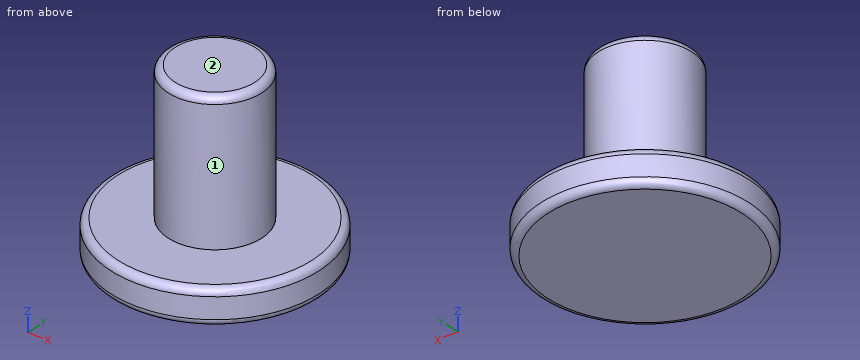
```python
from build123d import *

# Parameters (mm, degrees)
F0_R     = 6.75
F1_DEPTH = 25
F0_R_2   = 15
F2_DEPTH = 5
F3_R     = 1


with BuildPart() as f1:
    # F0 (on Top) → F1 (new body)
    with BuildSketch(Plane.XY):
        Circle(F0_R)
    extrude(amount=F1_DEPTH)

    # F0 (on Top) → F2 (join)
    with BuildSketch(Plane.XY):
        Circle(F0_R_2)
        Circle(F0_R, mode=Mode.SUBTRACT)
    extrude(amount=F2_DEPTH)

    # F3
    f3_edges = [f1.edges().sort_by_distance(p)[0] for p in [
        (-15, 0, 0),
        (-15, 0, 5),
        (-6.75, 0, 25),
    ]]
    fillet(f3_edges, radius=F3_R)


solid = f1.part
```
For this review, take the finished solid that the model builds, in its own axes (mm). Face numbers are marked on the shaded views. A direction names the side the tool comes from. Round coordinates to 2 decimals unless told otherwise and drop trailing zeros. Write each loop counter-clockwise with the first axis right and the second up, starting at its lowest first coordinate (ties: lowest second). Pieces come first, ordered by that corner, then holes. Notation, with made-up numbers: (7, 24) -> (13, 24) arc R30 ccw to (13, 58) -> close; hole circle Ø8 at (66.25, 58). An arc over 180 degrees is marked (long way). One line per question, with ' | ' between items. Start each with the question number.
1) For pin 1 Ø12 at (x, z) = (7.5, 18) entering from +Y; pin 2 Ø1 at (y, z) = (8.5, 17) entering from -X; pin 3 Ø12 at (x, z) = (-6, 20) entering from -Y; pin 4 Ø12 at (y, z) = (2, 15) entering from +X, all flat-tipped, find the tip position at first contact; note any pin that passes through.
2) Add section C-C (z = 18.5). Write out the cut boundary in (x, y).
3) Machinability: for the marked faces 1 and 2, which of the approach directions +Z, -Z, +X, -X, +Y, -Y give a long, thin tool a straight path to every point of the face, cutting with its end or side? Answer none if there is none.
4) Add section A-A (y = 0). Write out the cut boundary in (x, z).
5) Wall thickness on line 1 along Z through (x, y) = (11.25, -6.5); line 2 along Y through (x, z) = (0.25, 23); line 3 along Y through (x, z) = (-5.5, 5.25): over which ranges is each line inside the solid? List them lowest first.
Reported:
1) pin 1: stops at y = 6.58 | pin 2: passes through | pin 3: stops at y = -6.75 | pin 4: stops at x = 6.75
2) outline: circle Ø13.5 at (0, 0)
3) face 1: +Z | face 2: +Z, +X, -X, +Y, -Y
4) outline: (-15, 1) arc R1 ccw to (-14, 0) -> (14, 0) arc R1 ccw to (15, 1) -> (15, 4) arc R1 ccw to (14, 5) -> (6.75, 5) -> (6.75, 24) arc R1 ccw to (5.75, 25) -> (-5.75, 25) arc R1 ccw to (-6.75, 24) -> (-6.75, 5) -> (-14, 5) arc R1 ccw to (-15, 4) -> close
5) line 1: z = 0 to 5 | line 2: y = -6.75 to 6.75 | line 3: y = -3.91 to 3.91
